The model under review builds one solid part; all positions refer to its coordinate system, in mm. Face numbers are marked on the shaded views. Coordinates: 2 decimals unless noted, no trailing zeros. Loops run counter-clockwise (first coordinate to the right, second up) from the corner with the lowest first, then second, coordinate; pieces in that order, holes last. Notation, with made-up numbers: M 13.5,82.5 L 36.5,82.5 A9 ccw 36.5,98.5 Z; hole C -29,14.5 d11. An arc over 180 degrees is marked long. Return JSON: item names as keys, results as strings.
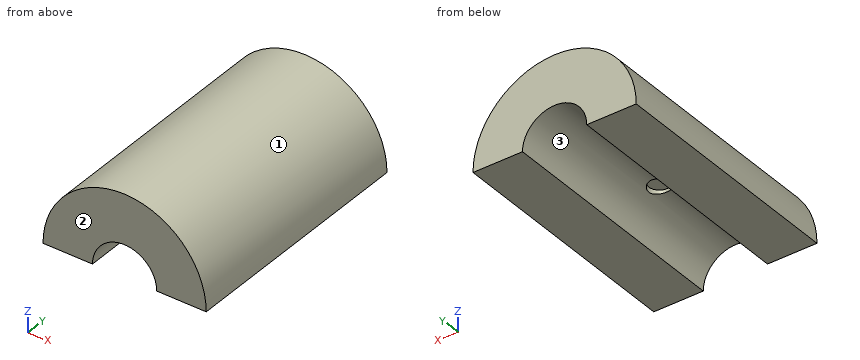
Autodesk Inventor part; units mm, degrees
ref_plane "YZ Plane" through (0, 0, 0) normal (1, 0, 0) x (0, 1, 0)
ref_plane "XZ Plane" through (0, 0, 0) normal (0, 1, 0) x (-1, 0, 0)
ref_plane "XY Plane" through (0, 0, 0) normal (0, 0, 1) x (1, 0, 0)
sketch "Sketch1" plane through (0, 0, 0) normal (0, 1, 0) x (-1, 0, 0)
  circle A0 centre (0, 0) radius 25.4
  circle A1 centre (0, 0) radius 10
  line L0 (-25.4, 0) -> (-10, 0)
  line L1 (10, 0) -> (25.4, 0)
  dimension "d0" = 50.8
  dimension "d1" = 20
extrude "Extrusion1" add sketch "Sketch1" along normal mid plane 76.2 contours L1 A1 L0 A0 picked at (-20.0206, 2.0262)
sketch "Sketch2" plane through (0, 0, 0) normal (0, 0, 1) x (1, 0, 0)
  circle A0 centre (0, -6) radius 3.25
  line L0 (46.8316, 0) -> (-44.45, 0)
  point P0 (0, 0)
  dimension "d4" = 6.5
  dimension "d6" = 6
extrude "Extrusion2" cut sketch "Sketch2" along normal blind 11
properties part number "Linear Actuatur piece 2"
1. The part is to be moulded in two halves that separate along X. For the marked faces 1, 2 and 3, say which applies: released by +X, released by -X, zero draft, split by the parting line, or undercut.
Check values:
{"face 1": "split by the parting line", "face 2": "zero draft", "face 3": "undercut"}
2. To check wall thickness, follow line 1 (Y direction, x = 0, z = 10.5); line 2 (X direction, y = -6, z = 10); line 3 (X direction, y = 18, z = 4.25). State the ranges of each line that lie inside material, in increasing order.
Check values:
{"line 1": "-38.1 to -9.25, -2.75 to 38.1", "line 2": "-23.35 to -3.25, 3.25 to 23.35", "line 3": "-25.04 to -9.05, 9.05 to 25.04"}
3. Add section D-D on z = 13. Give the boundary of the cut face in (x, y), plus the area to 3 significant figures.
Check values:
{"outline": "M -21.82,-38.1 L 21.82,-38.1 L 21.82,38.1 L -21.82,38.1 Z", "area": "3,330 mm²"}
4. Add section A-A on z = 5.5. Give the boundary of the cut face in (x, y), plus the area to 3 significant figures.
Check values:
{"outline": "M -24.8,-38.1 L -8.35,-38.1 L -8.35,38.1 L -24.8,38.1 Z; M 8.35,-38.1 L 24.8,-38.1 L 24.8,38.1 L 8.35,38.1 Z", "area": "2,510 mm²"}
5. Add section C-C on y = -6. Give the boundary of the cut face in (x, z).
Check values:
{"outline": "M -25.4,0 L -10,0 A10 cw -3.25,9.46 L -3.25,11 L 3.25,11 L 3.25,9.46 A10 cw 10,0 L 25.4,0 A25.4 ccw Z"}
6. Insertion check: pin 1 Ø10.5 at (x, y) = (0, -6) entering from +Z; pin 2 Ø3 at (x, y) = (-18, 21) entering from +Z; pin 3 Ø1 at (y, z) = (6, 19.5) entering from -X. Each pin has a flat end and moves straight along its axis. Give the tip position at first contact, or say it passes through.
Check values:
{"pin 1": "z = 25.4", "pin 2": "z = 19.31", "pin 3": "x = -16.86"}
7. Add section B-B on x = 0. Give the boundary of the cut face in (y, z), plus the area to 3 significant figures.
Check values:
{"outline": "M -38.1,10 L -9.25,10 L -9.25,11 L -2.75,11 L -2.75,10 L 38.1,10 L 38.1,25.4 L -38.1,25.4 Z", "area": "1,170 mm²"}
